Read the model definition and answer for the solid it produces. Units are mm, in the model's axes. Round coordinates to 2 decimals unless told otherwise and drop trailing zeros. Write each loop counter-clockwise with the first axis right and the second up, starting at its lowest first coordinate (ties: lowest second). Pieces come first, ordered by that corner, then holes. Notation, with made-up numbers: (41, 10) -> (81, 10) arc R15 cw to (81, 34) -> close; hole circle Ø7 at (-40, 7.25). An arc over 180 degrees is marked (long way). Return JSON: item names as keys, results as strings.
from build123d import *

# Parameters (mm, degrees)
F0_W     = 88.9
F0_H     = 12.7
F0_R     = 3.2385
F1_DEPTH = 6.35
F3_D     = 2.7051


with BuildPart() as f1:
    # F0 (on Front) → F1 (new body)
    with BuildSketch(Plane.XZ):
        Rectangle(F0_W, F0_H)
        with Locations((-39.37, 1.27)):
            Circle(F0_R, mode=Mode.SUBTRACT)
    extrude(amount=F1_DEPTH)

    # F3 (through all)
    with Locations(Plane(origin=(0, 0, -6.35), x_dir=(1, 0, 0), z_dir=(0, 0, -1))):
        with Locations((-25.4, 3.175), (38.1, 3.175)):
            Hole(F3_D / 2)


solid = f1.part
Item 1: Section D-D (x = -25.4) is taken. Give the vertices of the cut face in (y, z).
Worked answers:
{"outline": "(-6.35, -6.35) -> (-4.53, -6.35) -> (-4.53, 6.35) -> (-6.35, 6.35) -> close; (-1.82, -6.35) -> (0, -6.35) -> (0, 6.35) -> (-1.82, 6.35) -> close"}
Item 2: A flat-ended cylindrical pin translates along its axis: pin 1 (2 mm diameter, centred on x = 38.1, y = -3.175, fed in from +Z). Find the tip coordinate at first contact, or state that the pin passes through.
Worked answers:
{"pin 1": "passes through"}
Item 3: Section A-A (x = -39.37) is taken. Give the vertices of the cut face in (y, z), then the cut area to 3 significant figures.
Worked answers:
{"outline": "(-6.35, -6.35) -> (0, -6.35) -> (0, -1.97) -> (-6.35, -1.97) -> close; (-6.35, 4.51) -> (0, 4.51) -> (0, 6.35) -> (-6.35, 6.35) -> close", "area": "39.5 mm2"}
Item 4: Section B-B (z = 2.5) is taken. Give the vertices of the cut face in (x, y) (3 decimals).
Worked answers:
{"outline": "(-44.45, -6.35) -> (-42.366, -6.35) -> (-42.366, 0) -> (-44.45, 0) -> close; (-36.374, -6.35) -> (44.45, -6.35) -> (44.45, 0) -> (-36.374, 0) -> close; hole circle Ø2.705 at (-25.4, -3.175); hole circle Ø2.705 at (38.1, -3.175)"}
Item 5: Straight lines are drawn through the part: L1, parallel to X at y = -4, z = -2.75; L2, parallel to X at y = -4.25, z = 5; L3, parallel to Y at x = -25.4, z = 3.25. For each, find the intervals that lie inside material, in ascending order. Write a range as [from, to].
Worked answers:
{"L1": "x = [-44.45, -26.47], [-24.33, 37.03], [39.17, 44.45]", "L2": "x = [-44.45, -26.22], [-24.58, 37.28], [38.92, 44.45]", "L3": "y = [-6.35, -4.53], [-1.82, 0]"}
Item 6: For a pull along X with two mould halves and no side action, classify faces 1 (the flat face through (44.45, -3, 0)), 2 (the cylindrical face through (36.81, -3.58, 0.09)), 3 (the flat face through (-44.45, -3, 0)) as released by +X, released by -X, zero draft, split by the parting line, or undercut.
Worked answers:
{"face 1": "released by +X", "face 2": "undercut", "face 3": "released by -X"}
Item 7: Section C-C (y = -1) is taken. Give the vertices of the cut face in (x, z).
Worked answers:
{"outline": "(-44.45, -6.35) -> (44.45, -6.35) -> (44.45, 6.35) -> (-44.45, 6.35) -> close; hole circle Ø6.48 at (-39.37, 1.27)"}
